Read the model definition and answer for the solid it produces. Units are mm, in the model's axes. A direction names the side the tool comes from. Coordinates: 2 decimals unless noted, no trailing zeros. Loops run counter-clockwise (first coordinate to the right, second up) from the corner with the lowest first, then second, coordinate; pieces in that order, holes last. Notation, with made-up numbers: M 84,53.5 L 137,53.5 A28 cw 137,77.5 Z; hole C 64,41 d9. An arc over 180 degrees is marked long. Put each result on its own line as item: value.
from build123d import *

# Parameters (mm, degrees)
EXTRUDE_1_DEPTH         = 30
EXTRUDE_1_DEPTH_BACK    = 40
SKETCH_2_W              = 49
SKETCH_2_H              = 24
SKETCH_2_W_2            = 43
SKETCH_2_H_2            = 18
EXTRUDE_1_2_DEPTH       = 6
SKETCH_1_3_W            = 20
SKETCH_1_3_H            = 8
EXTRUDE_2_DEPTH         = 24.5
CUT_EXTRUDE_1_DEPTH     = 25
RIB_1_REACH             = 58.032
SKETCH_4_WALLS_W        = 145.49538697
SKETCH_4_WALLS_H        = 3
RIB_2_REACH             = 65.649
SKETCH_6_WALLS_W        = 3
SKETCH_6_WALLS_H        = 137.784142328
CUT_EXTRUDE_START       = -12
CUT_EXTRUDE_2_OUTLINE_R = 4
CUT_EXTRUDE_2_DEPTH     = 3
FILLET_1_R              = 1
SKETCH_7_R              = 5
CUT_EXTRUDE_4_DEPTH     = 2


# Read off the part's stored shape, not the designer's step: the extrude step
with BuildPart() as part:
    # Sketch 2 → Extrude 1 (new, two sides: drawn at the far end of the back side and taken through both)
    with BuildSketch(Plane(origin=(0, 0, 0), x_dir=(0, 0, -1), z_dir=(1, 0, 0)).offset(-EXTRUDE_1_DEPTH_BACK)):
        with Locations((0, -21)):
            Rectangle(SKETCH_2_W, SKETCH_2_H)
        with Locations((0, -21)):
            Rectangle(SKETCH_2_W_2, SKETCH_2_H_2, mode=Mode.SUBTRACT)
    extrude(amount=EXTRUDE_1_DEPTH + EXTRUDE_1_DEPTH_BACK)



with BuildPart() as body_2:
    # Sketch 1 → Extrude 1 2 (new, symmetric)
    with BuildSketch(Plane.XY):
        Polygon((-10, 19.5), (-10, 0), (10, 0), (10, 8), (10, 19.5), align=None)
    extrude(amount=EXTRUDE_1_2_DEPTH, both=True)


with BuildPart() as part_1:
    add(part.part)

    add(body_2.part)  # Extrude 2 merges body 2
    # Sketch 1_3 → Extrude 2 (add, symmetric)
    with BuildSketch(Plane.XY):
        Polygon((10, 0), (-10, 0), (-10, -12), (10, -12), (30, -12), (30, 0), align=None)
        with Locations((20, 4)):
            Rectangle(SKETCH_1_3_W, SKETCH_1_3_H)
    extrude(amount=EXTRUDE_2_DEPTH, both=True)

    # Sketch 1_4 → Cut-Extrude 1 (cut, symmetric)
    with BuildSketch(Plane.XY):
        Polygon((30, -12), (10, -12), (-11, -33), (30, -33), align=None)
    extrude(amount=CUT_EXTRUDE_1_DEPTH, both=True, mode=Mode.SUBTRACT)

    # Sketch 4 walls → Rib 1 (add, up to next)
    with BuildSketch(Plane(origin=(0.4400978, -2.93398533, 0), x_dir=(0.9889363528682976, 0.14834045293024445, 0), z_dir=(-0.14834045293024445, 0.9889363528682976, 0)), mode=Mode.PRIVATE) as rib_1_sk1:
        with Locations((-25.177107795, -12.5)):
            Rectangle(SKETCH_4_WALLS_W, SKETCH_4_WALLS_H)
    rib_1_tool1 = extrude(rib_1_sk1.sketch, amount=-RIB_1_REACH, mode=Mode.PRIVATE) - part_1.part
    # Sketch 4 walls → Rib 1 (add, up to next)
    with BuildSketch(Plane(origin=(0.4400978, -2.93398533, 0), x_dir=(0.9889363528682976, 0.14834045293024445, 0), z_dir=(-0.14834045293024445, 0.9889363528682976, 0)), mode=Mode.PRIVATE) as rib_1_sk2:
        with Locations((-25.177107795, 12.5)):
            Rectangle(SKETCH_4_WALLS_W, SKETCH_4_WALLS_H)
    rib_1_tool2 = extrude(rib_1_sk2.sketch, amount=-RIB_1_REACH, mode=Mode.PRIVATE) - part_1.part
    add(rib_1_tool1.solids().sort_by_distance((-24.458459359, -6.668768904, 12.5))[0])
    add(rib_1_tool2.solids().sort_by_distance((-24.458459359, -6.668768904, -12.5))[0])

    # Sketch 6 walls → Rib 2 (add, up to next)
    with BuildSketch(Plane(origin=(0, 6, -6), x_dir=(1, 0, 0), z_dir=(0, 0.7071067811865477, -0.7071067811865474)), mode=Mode.PRIVATE) as rib_2_sk1:
        with Locations((0, 4.242640687)):
            Rectangle(SKETCH_6_WALLS_W, SKETCH_6_WALLS_H)
    rib_2_tool1 = extrude(rib_2_sk1.sketch, amount=-RIB_2_REACH, mode=Mode.PRIVATE) - part_1.part
    rib_2 = rib_2_tool1.solids().sort_by_distance((0, 3, -9))[0]
    add(rib_2)

    # Mirror 1: Rib 2 across plane
    add(rib_2.mirror(Plane.XY))

    # Cut-Extrude 2 outline → Cut-Extrude 2 (cut)
    with BuildSketch(Plane(origin=(0, 0, 0), x_dir=(1, 0, 0), z_dir=(0, 1, 0)).offset(CUT_EXTRUDE_START)):
        with Locations((-29, 0)):
            Circle(CUT_EXTRUDE_2_OUTLINE_R)
    extrude(amount=CUT_EXTRUDE_2_DEPTH, mode=Mode.SUBTRACT)

    # Fillet 1
    fillet_1_edges = [part_1.edges().sort_by_distance(p)[0] for p in [
        (30, -2, 24.5),
        (30, -12, 0),
        (20, 8, -24.5),
        (30, 8, 0),
        (10, 8, 15.25),
        (20, 8, 24.5),
        (-25.5, -33, 24.5),
        (-25, -9, 24.5),
        (-25, -9, -24.5),
        (-25.5, -33, -24.5),
        (30, -2, -24.5),
        (20, -12, 24.5),
        (20, -12, -24.5),
    ]]
    fillet(fillet_1_edges, radius=FILLET_1_R)

    # Sketch 7 → Cut-Extrude 4 (cut)
    with BuildSketch(Plane(origin=(0, 19.5, 0), x_dir=(1, 0, 0), z_dir=(0, 1, 0))):
        with Locations(Location((0, 0, 0), (0, 0, 270))):
            Circle(SKETCH_7_R)
    extrude(amount=-CUT_EXTRUDE_4_DEPTH, mode=Mode.SUBTRACT)


solid = part_1.part
1) Given pin 1 Ø2 at (y, z) = (2, 18) entering from -X; pin 2 Ø10.5 at (x, z) = (-24, -20.5) entering from +Y; pin 3 Ø20.5 at (x, z) = (-0.5, -12.5) entering from +Y; pin 4 Ø6 at (x, y) = (0, 12) entering from +Z, each flat-ended and moving along its own axis, determine where each tip first touches the part or whether it passes through.
Answer list:
pin 1: stops at x = 10
pin 2: stops at y = -9
pin 3: stops at y = 19.5
pin 4: stops at z = 6
2) Find section A-A, the plane y = -23. Write down the section's boundary in (x, z), plus the area to 3 significant figures.
Answer list:
outline: M -40,-24.5 L -1,-24.5 L -1,-21.5 L -40,-21.5 Z; M -40,21.5 L -1,21.5 L -1,24.5 L -40,24.5 Z
area: 234 mm^2
3) Find section B-B, the plane z = -9.5. Write down the section's boundary in (x, y).
Answer list:
outline: M -40,-33 L -11,-33 L -8,-30 L -40,-30 Z; M -40,-12 L 29,-12 A1 ccw 30,-11 L 30,7 A1 ccw 29,8 L 10,8 L 10,0 L 1.5,0 L 1.5,2.5 L -1.5,2.5 L -1.5,0 L -10,0 L -10,-9 L -40,-9 Z
4) Find section D-D, the plane z = 0. Write down the section's boundary in (x, y), plus the area to 3 significant figures.
Answer list:
outline: M -40,-33 L -11,-33 L -8,-30 L -40,-30 Z; M -40,-12 L -33,-12 L -33,-9 L -40,-9 Z; M -25,-12 L 29,-12 A1 ccw 30,-11 L 30,7 A1 ccw 29,8 L 10,8 L 10,19.5 L 5,19.5 L 5,17.5 L -5,17.5 L -5,19.5 L -10,19.5 L -10,-9 L -25,-9 Z
area: 1,170 mm^2
5) Find section C-C, the plane x = -16. Write down the section's boundary in (y, z), plus the area to 3 significant figures.
Answer list:
outline: M -33,-23.5 A1 ccw -32,-24.5 L -10,-24.5 A1 ccw -9,-23.5 L -9,-14 L -5.4,-14 L -5.4,-11 L -9,-11 L -9,11 L -5.4,11 L -5.4,14 L -9,14 L -9,23.5 A1 ccw -10,24.5 L -32,24.5 A1 ccw -33,23.5 Z; hole M -30,-21.5 L -12,-21.5 L -12,21.5 L -30,21.5 Z
area: 423 mm^2
6) Which of the six approach directions +Z, -Z, +X, -X, +Y, -Y give full straight-line access (tool end or side, diameter ignored) to faces 1 (the cylindrical face through (-32.2, -10.5, 2.4)), 2 (the flat face through (19, 8, 0)), 3 (the flat face through (-25, -9, -19)), 4 (the flat face through (0, 10, 6))?
Answer list:
face 1: +Y
face 2: +Z, -Z, +X, +Y
face 3: -Z, -X, +Y
face 4: +Z, +Y
7) Determine the mould class of faces 5 (the flat face through (-22, -8, 11)), 6 (the flat face through (-9, -31, 2)), 7 (the flat face through (0, 0, 15)), 8 (the flat face through (-24, -30, 0)) for opening direction Y: released by +Y, released by -Y, zero draft, split by the parting line, or undercut.
Answer list:
face 5: zero draft
face 6: released by -Y
face 7: released by +Y
face 8: undercut
8) Straight lines are drawn through the part: line 1 (X direction, y = -10.15, z = 0); line 2 (Y direction, x = -11, z = 7.5); line 3 (Z direction, x = -29, y = -10). For each, find the intervals that lie inside material, in ascending order. Write a range as [from, to].
Answer list:
line 1: x = [-40, -33], [-25, 30]
line 2: y = [-33, -30], [-12, -9]
line 3: z = [-24.5, -4], [4, 24.5]
